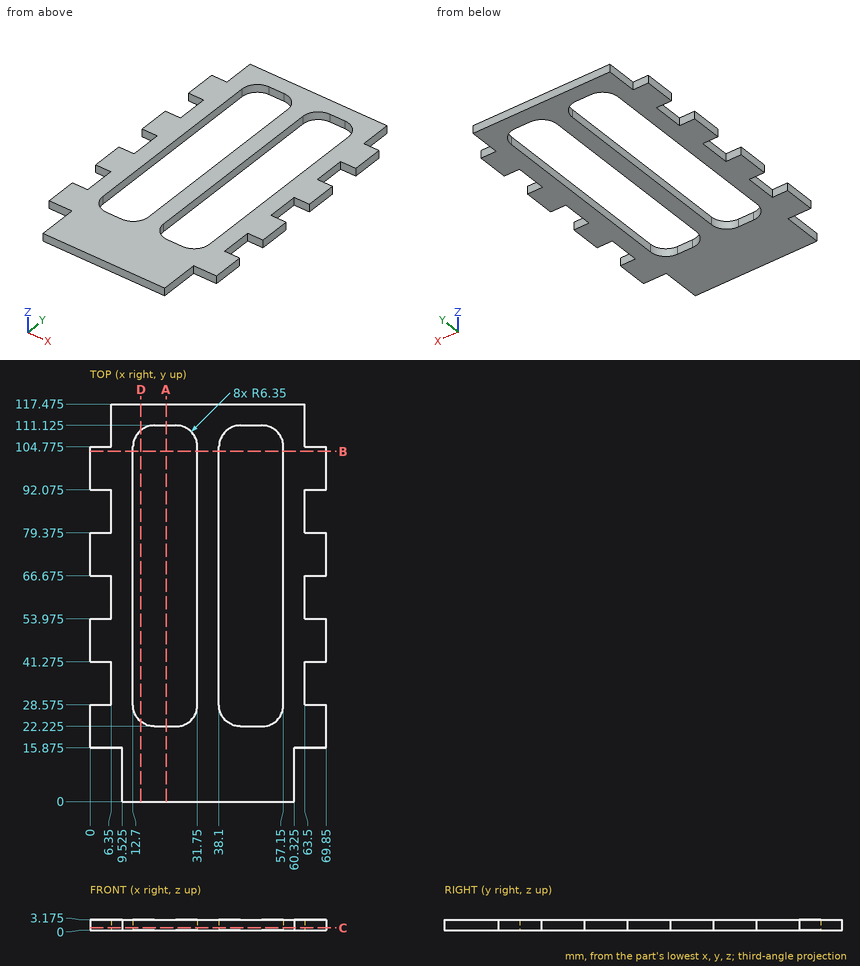
Input: dimensioned drawing with shaded views. Units: mm. Origin: part minimum x, y, z. Coordinates: 2 decimals unless noted, no trailing zeros. Loops run counter-clockwise (first coordinate to the right, second up) from the corner with the lowest first, then second, coordinate; pieces in that order, holes last. Notation, with made-up numbers: M 73.25,17 L 97.25,17 A9 ccw 97.25,34 Z; hole C -36,0.5 d2. An arc over 180 degrees is marked long. One line per item, written item: value.
(1) Section D-D (x = 15). Output: boundary loops of the cut face in (y, z) (3 decimals).
Filled in:
outline: M 0,0 L 23.684,0 L 23.684,3.175 L 0,3.175 Z; M 109.666,0 L 117.475,0 L 117.475,3.175 L 109.666,3.175 Z
(2) Section A-A (x = 22.5). Output: boundary loops of the cut face in (y, z) (3 decimals).
Filled in:
outline: M 0,0 L 22.225,0 L 22.225,3.175 L 0,3.175 Z; M 111.125,0 L 117.475,0 L 117.475,3.175 L 111.125,3.175 Z
(3) Section C-C (z = 0.7). Give the number of separate pieces and of enclosed holes in the cut face, and give its area (3 significant figures).
Filled in:
separate pieces: 1
enclosed holes: 2
area: 3,940 mm^2
(4) Pin query (flat end, axial travel): pin 1 (1 mm diameter, centred on x = 66, z = 1.5, fed in from -Y) (3 decimals); pin 2 (1.6 mm diameter, centred on y = 4.5, z = 1, fed in from +X) (3 decimals). Return the tip coordinate at first contact, or that it passes through.
Filled in:
pin 1: y = 15.875
pin 2: x = 60.325
(5) Line query: line 1 along X through (y, z) = (76, 2.3); line 2 along X through (y, z) = (62, 2.6); line 3 along Y through (x, z) = (50, 2.35) (3 decimals). Output: solid intervals per line, ascending. Write a range as from..to.
Filled in:
line 1: 0..12.7, 31.75..38.1, 57.15..69.85
line 2: 6.35..12.7, 31.75..38.1, 57.15..63.5
line 3: 0..22.225, 111.125..117.475
(6) Section B-B (y = 103.5). Output: boundary loops of the cut face in (x, z) (3 decimals).
Filled in:
outline: M 0,0 L 12.7,0 L 12.7,3.175 L 0,3.175 Z; M 31.75,0 L 38.1,0 L 38.1,3.175 L 31.75,3.175 Z; M 57.15,0 L 69.85,0 L 69.85,3.175 L 57.15,3.175 Z
